Part print with two shaded views. Sizes in mm from the minimum x, y, z corner. A direction names the side the tool comes from. Give positions to 0.01 mm unless a question says otherwise; leave off trailing zeros. Order: outer loops, then holes, each group sorted by start corner. A loop starts at its lowest first (then second) coordinate and runs counter-clockwise, first axis right, second up. Notation, with made-up numbers: M 21.5,37 L 50.5,37 A15 ccw 50.5,63 Z; hole C 42.25,79 d4. An arc over 180 degrees is marked long. Return JSON: item names as keys, results as strings.
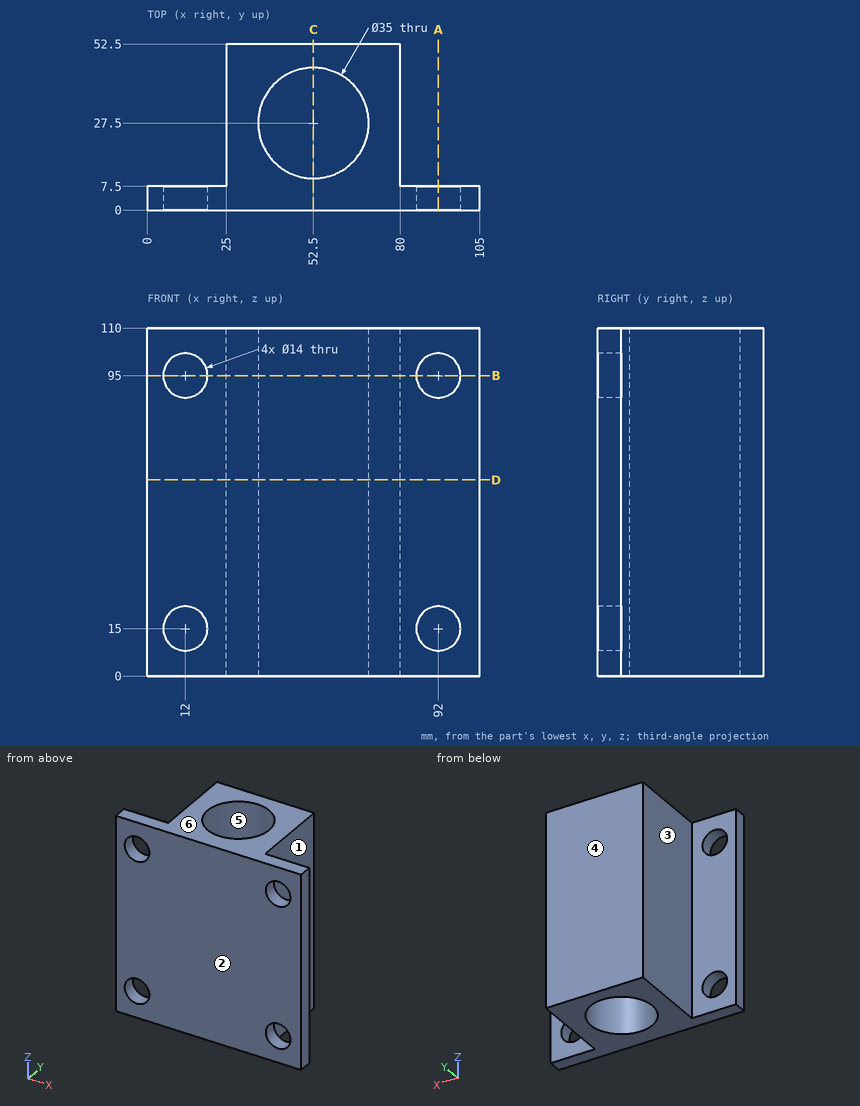
Q1. Band-saw the part on A-A (x = 92). Give the cut face in (y, z), then the cut area to 3 significant figures.
Established:
{"outline": "M 0,0 L 7.5,0 L 7.5,8 L 0,8 Z; M 0,22 L 7.5,22 L 7.5,88 L 0,88 Z; M 0,102 L 7.5,102 L 7.5,110 L 0,110 Z", "area": "615 mm²"}
Q2. Pin check, flat tips, straight feed: pin 1 (20 mm diameter, centred on x = 9.5, z = 63.5, fed in from +Y); pin 2 (6 mm diameter, centred on x = 91.5, z = 73, fed in from -Y); pin 3 (13.5 mm diameter, centred on y = 38, z = 59.5, fed in from +X); pin 4 (13.5 mm diameter, centred on y = 33.5, z = 39.5, fed in from -X). Stop position of each tip, or through.
Established:
{"pin 1": "stops at y = 7.5", "pin 2": "stops at y = 0", "pin 3": "stops at x = 80", "pin 4": "stops at x = 25"}
Q3. Probe line 1 along Z through (x, y) = (12, 2.75); line 2 along X through (y, z) = (28.5, 65); line 3 along X through (y, z) = (49.5, 93). List the from-to ranges inside material, lowest first.
Established:
{"line 1": "z = 0 to 8, 22 to 88, 102 to 110", "line 2": "x = 25 to 35.03, 69.97 to 80", "line 3": "x = 25 to 80"}
Q4. Band-saw the part on C-C (x = 52.5). Give the cut face in (y, z).
Established:
{"outline": "M 0,0 L 10,0 L 10,110 L 0,110 Z; M 45,0 L 52.5,0 L 52.5,110 L 45,110 Z"}
Q5. Two-plate mould, pull along Y, no slides. Class the marked faces 4, 5 and 6: +Y half, -Y half, draft (parallel to the pull), parting line (faces both ways), or undercut.
Established:
{"face 4": "+Y half", "face 5": "undercut", "face 6": "draft"}
Q6. 3-axis set-ups, long thin cutter, end or side, ignore diameter. For the marked faces 1, 2 and 3: which of +Z, -Z, +X, -X, +Y, -Y reach the whole face in a straight line?
Established:
{"face 1": "+Z, -Z, +X, +Y", "face 2": "+Z, -Z, +X, -X, -Y", "face 3": "+Z, -Z, -X, +Y"}
Q7. Band-saw the part on B-B (z = 95). Give the cut face in (x, y).
Established:
{"outline": "M 0,0 L 5,0 L 5,7.5 L 0,7.5 Z; M 19,0 L 85,0 L 85,7.5 L 80,7.5 L 80,52.5 L 25,52.5 L 25,7.5 L 19,7.5 Z; M 99,0 L 105,0 L 105,7.5 L 99,7.5 Z; hole C 52.5,27.5 d35"}
Q8. Band-saw the part on D-D (z = 62). Give the cut face in (x, y), then the cut area to 3 significant figures.
Established:
{"outline": "M 0,0 L 105,0 L 105,7.5 L 80,7.5 L 80,52.5 L 25,52.5 L 25,7.5 L 0,7.5 Z; hole C 52.5,27.5 d35", "area": "2,300 mm²"}
